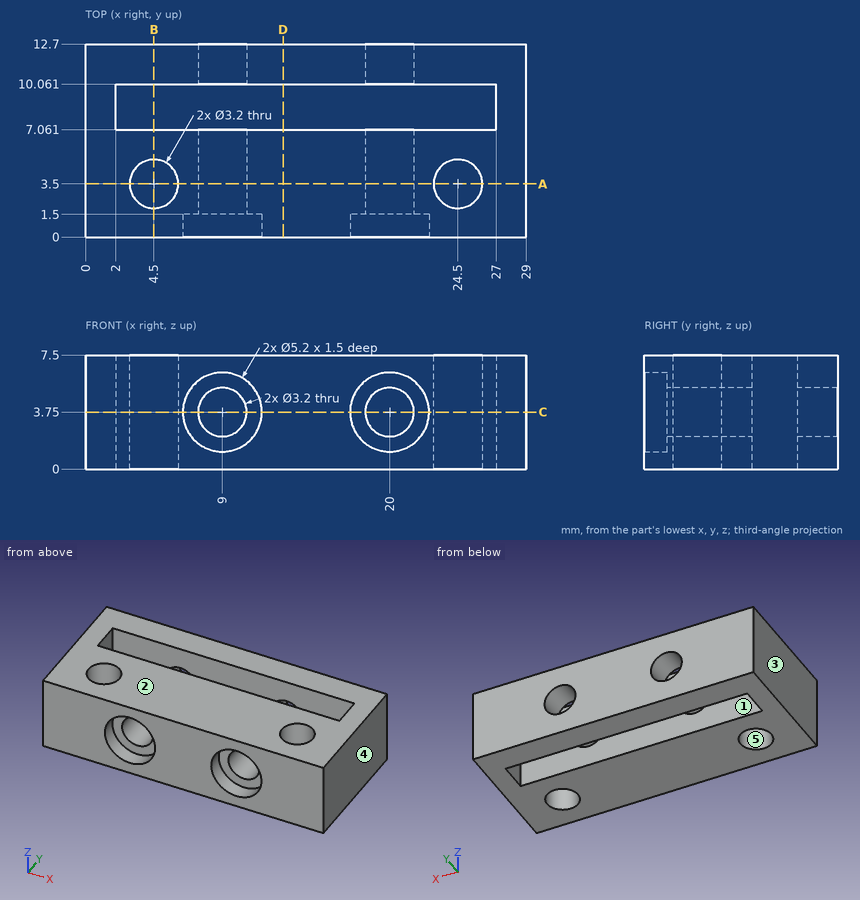
For this review, use the dimensioned drawing (mm, ordinates from the lowest corner) and the shaded views. A direction names the side the tool comes from. Give positions to 0.01 mm unless a question says otherwise; leave off trailing zeros. Write each loop counter-clockwise with the first axis right and the second up, starting at its lowest first coordinate (ties: lowest second). Pieces come first, ordered by that corner, then holes. Notation, with made-up numbers: M 58,-16.5 L 116,-16.5 A4 cw 116,-11.5 Z; hole C 41.25,86 d8. An arc over 180 degrees is marked long. Answer as a JSON object with one key per item and string values. Group by question number.
Item 1: Draft analysis for pull direction X (two halves, no side actions). For the marked faces 3, 4 and 5, state which applies: +X half, -X half, draft (parallel to the pull), parting line (faces both ways), or undercut.
Item 2: Consider section A-A on y = 3.5. Write out the cut boundary in (x, z).
Item 3: Tool access review of the marked faces 1 and 2: name each direction out of +Z, -Z, +X, -X, +Y, -Y from which nothing blocks a thin tool from reaching the whole face with its end or side.
Item 4: Consider section B-B on x = 4.5. Write out the cut boundary in (y, z).
Item 5: Consider section D-D on x = 13. Write out the cut boundary in (y, z).
Item 6: For probe 1 along X at (y, z) = (12.05, 3.75); probe 2 along X at (y, z) = (1, 3.75); probe 3 along X at (y, z) = (8.75, 6.5), list the stretches that pass through material, from the lowest coordinate up. Write a range as [from, to].
Item 7: For pin 1 Ø2 at (x, y) = (24, 3.5) entering from +Z; pin 2 Ø4.5 at (x, z) = (9, 3.75) entering from -Y, all flat-tipped, find the tip position at first contact; note any pin that passes through.
Item 8: Consider section C-C on z = 3.75. Count the separate pieces of the cut face and the enclosed holes in it, plus the area to 3 significant figures.
Check result:
{
 "1": {"face 3": "-X half", "face 4": "+X half", "face 5": "undercut"},
 "2": {"outline": "M 0,0 L 2.9,0 L 2.9,7.5 L 0,7.5 Z; M 6.1,0 L 22.9,0 L 22.9,7.5 L 6.1,7.5 Z; M 26.1,0 L 29,0 L 29,7.5 L 26.1,7.5 Z; hole C 9,3.75 d3.2; hole C 20,3.75 d3.2"},
 "3": {"face 1": "+Z, -Z", "face 2": "+Z, +X, -X, +Y, -Y"},
 "4": {"outline": "M 0,0 L 1.9,0 L 1.9,7.5 L 0,7.5 Z; M 5.1,0 L 7.06,0 L 7.06,7.5 L 5.1,7.5 Z; M 10.06,0 L 12.7,0 L 12.7,7.5 L 10.06,7.5 Z"},
 "5": {"outline": "M 0,0 L 7.06,0 L 7.06,7.5 L 0,7.5 Z; M 10.06,0 L 12.7,0 L 12.7,7.5 L 10.06,7.5 Z"},
 "6": {"probe 1": "x = [0, 7.4], [10.6, 18.4], [21.6, 29]", "probe 2": "x = [0, 6.4], [11.6, 17.4], [22.6, 29]", "probe 3": "x = [0, 2], [27, 29]"},
 "7": {"pin 1": "passes through", "pin 2": "stops at y = 1.5"},
 "8": {"separate pieces": "4", "enclosed holes": "2", "area": "209 mm^2"}
}
